The figure shows three views and two pictorial views of one solid part (mm, origin at its lowest corner). Answer the questions. Coordinates: 2 decimals unless noted, no trailing zeros. Order: outer loops, then holes, each group sorted by start corner. A loop starts at its lowest first (then second) coordinate and runs counter-clockwise, first axis right, second up. Notation, with made-up numbers: (-34.5, 76.5) - (3.5, 76.5) arc R17 cw to (3.5, 86.5) - close; hole circle Ø2 at (28, -9.75). An arc over 180 degrees is marked (long way). Use one line per item in the form item = value.
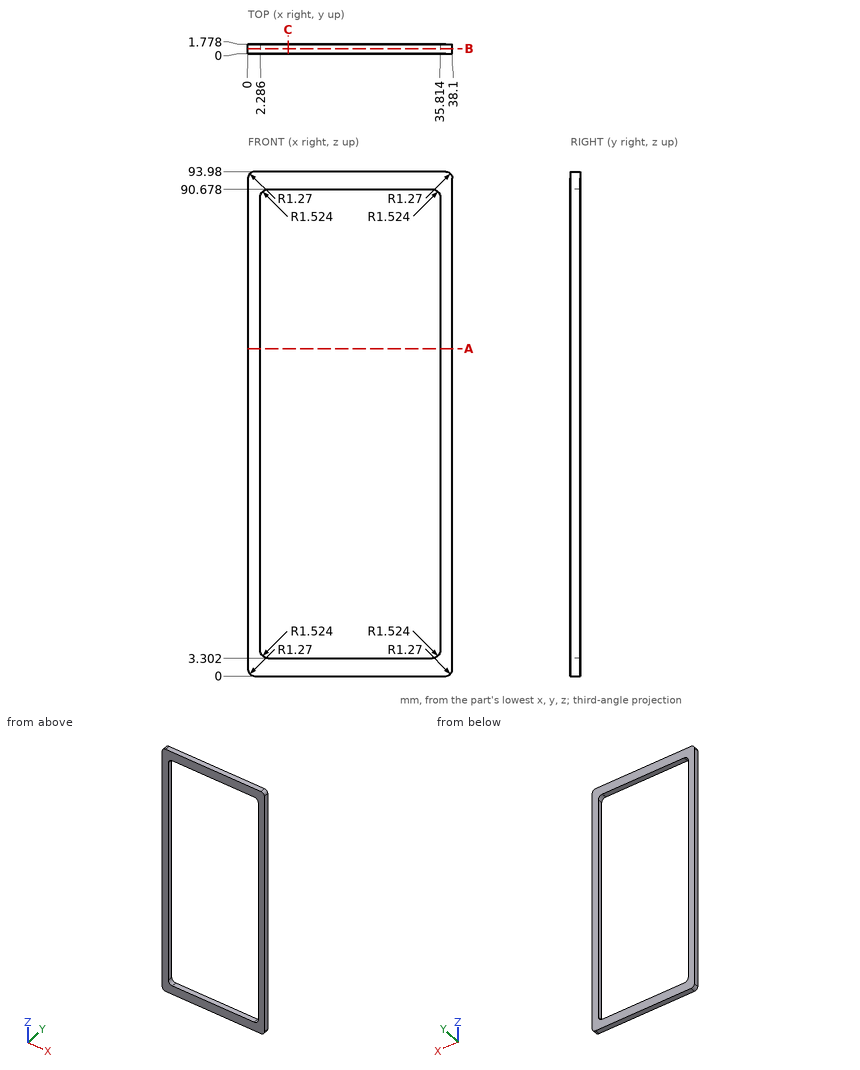
(1) Given pin 1 Ø0.5 at (x, y) = (13, 0.5) entering from -Z, flat-ended and moving along its own axis, determine where the tip first touches the part or whether it passes through.
Answer list:
pin_1 = 0
(2) Section A-A, the plane z = 61 is taken. Write down the section's boundary in (x, y), then the cut area to 3 significant figures.
Answer list:
outline = (0, 0) - (2.29, 0) - (2.29, 1.78) - (0, 1.78) - close; (35.81, 0) - (38.1, 0) - (38.1, 1.78) - (35.81, 1.78) - close
area = 8.13 mm2
(3) Straight lines are drawn through the part: L1, parallel to X at y = 0.15, z = 74; L2, parallel to Z at x = 19, y = 0.55. For each, find the intervals that lie inside material, in ascending order.
Answer list:
L1 = 0 to 2.29, 35.81 to 38.1
L2 = 0 to 3.3, 90.68 to 93.98
(4) Section C-C, the plane x = 7.5 is taken. Write down the section's boundary in (y, z).
Answer list:
outline = (0, 0) - (1.78, 0) - (1.78, 3.3) - (0, 3.3) - close; (0, 90.68) - (1.78, 90.68) - (1.78, 93.98) - (0, 93.98) - close
(5) Section B-B, the plane y = 0.9 is taken. Write down the section's boundary in (x, z), then the cut area to 3 significant figures.
Answer list:
outline = (0, 1.27) arc R1.27 ccw to (1.27, 0) - (36.83, 0) arc R1.27 ccw to (38.1, 1.27) - (38.1, 92.71) arc R1.27 ccw to (36.83, 93.98) - (1.27, 93.98) arc R1.27 ccw to (0, 92.71) - close; hole (2.29, 4.83) arc R1.52 ccw to (3.81, 3.3) - (34.29, 3.3) arc R1.52 ccw to (35.81, 4.83) - (35.81, 89.15) arc R1.52 ccw to (34.29, 90.68) - (3.81, 90.68) arc R1.52 ccw to (2.29, 89.15) - close
area = 652 mm2
